Read the model definition and answer for the solid it produces. Units are mm, in the model's axes. A direction names the side the tool comes from. Round coordinates to 2 decimals unless told otherwise and drop trailing zeros. Order: outer loops, then holes, each group sorted by start corner. A loop starts at its lowest first (then second) coordinate and runs counter-clockwise, first axis right, second up. Notation, with made-up numbers: M 46,82.5 L 85,82.5 A32 ccw 85,116.5 Z; hole C 32.5,81.5 d2. An arc over 180 degrees is marked long. Use one line per item in the form item = value. Start each with the question number.
from build123d import *

# Parameters (mm, degrees)
SKETCH_3_W             = 8
SKETCH_3_H             = 16.823898374
CUT_EXTRUDE_1_DEPTH    = 10
HOLE_WIZARD_M4_1_D     = 3.3
HOLE_WIZARD_M4_1_DEPTH = 11.5
HOLE_WIZARD_M4_1_TIP   = 0.991420021
SKETCH_5_OUTSIDE_W     = 23.696
SKETCH_5_OUTSIDE_H     = 27.696
SKETCH_5_OUTSIDE_R     = 7.77784742
CUT_EXTRUDE_2_DEPTH    = 10


with BuildPart() as part:
    # 草图2 → 旋转1 (revolve)
    with BuildSketch(Plane(origin=(0, 0, 0), x_dir=(0, 0, -1), z_dir=(1, 0, 0))):
        Polygon((0, 0), (0, 4), (15, 4), (15, 9), (21, 9), (21, 4), (31, 4), (31, 0), align=None)
    revolve(axis=Axis((0, 0, 0), (0, 0, -1)))

    # 草图3 → 切除-拉伸1 (cut)
    with BuildSketch(Plane.XY.offset(-15)):
        with Locations((-11, -0.026043186)):
            Rectangle(SKETCH_3_W, SKETCH_3_H)
        with Locations((11, -0.026043186)):
            Rectangle(SKETCH_3_W, SKETCH_3_H)
    extrude(amount=-CUT_EXTRUDE_1_DEPTH, mode=Mode.SUBTRACT)

    # M4 螺纹孔1
    with Locations(Plane(origin=(0, 0, -31), x_dir=(-1, 0, 0), z_dir=(0, 0, -1))):
        with Locations((0, 0)):
            Hole(HOLE_WIZARD_M4_1_D / 2, depth=HOLE_WIZARD_M4_1_DEPTH)
            with Locations((0, 0, -(HOLE_WIZARD_M4_1_DEPTH + HOLE_WIZARD_M4_1_TIP / 2))):  # 118° drill point
                Cone(0, HOLE_WIZARD_M4_1_D / 2, HOLE_WIZARD_M4_1_TIP, mode=Mode.SUBTRACT)

    # 草图5 outside → 切除-拉伸2 (cut)
    with BuildSketch(Plane(origin=(0, 0, -21), x_dir=(-1, 0, 0), z_dir=(0, 0, -1))):
        Rectangle(SKETCH_5_OUTSIDE_W, SKETCH_5_OUTSIDE_H)
        Circle(SKETCH_5_OUTSIDE_R, mode=Mode.SUBTRACT)
    extrude(amount=-CUT_EXTRUDE_2_DEPTH, mode=Mode.SUBTRACT)


solid = part.part
Item 1: For a pull along Y with two mould halves and no side action, classify faces 1 (the conical face through (0.1, -0.3, -18.7)), 2 (the cylindrical face through (0.122, -7.777, -18.042)), 3 (the cylindrical face through (-3.905, -0.867, -7.605)) as pulls with the +Y half, pulls with the -Y half, needs draft (parallel to the pull), parting line crosses it, or undercut.
Item 2: Section B-B (x = 3.25) is taken. Write down the section's boundary in (y, z).
Item 3: Section A-A (z = -24) is taken. Write down the section's boundary in (x, y), and give its area (3 significant figures).
Item 4: Find the intervals of material crossed by L1, parallel to X at y = 0, z = -24.5; L2, parallel to Z at x = 4, y = -2.25; L3, parallel to Y at x = 0.5, z = -24, in increasing order. Write a range as [from, to].
Item 5: Section D-D (y = 6.75) is taken. Write down the section's boundary in (x, z).
Item 6: Given P1, Ø5, axis at x = -3, z = -27, coming from the -Y side; P2, Ø1, axis at x = 5, y = 1.5, coming from the -Z side; P3, Ø1.5, axis at y = 4, z = -26, coming from the +X side, each flat-ended and moving along its own axis, determine where each tip first touches the part or whether it passes through.
Item 7: Section C-C (z = -17) is taken. Write down the section's boundary in (x, y).
Item 8: A tool of negligible diameter and unlimited length cuts with its end or side. For faces 4 (the flat face through (0, 2, -31)), 5 (the flat face through (3, 4, -15)), 6 (the cylindrical face through (-3.905, -0.867, -26.07)), from which of +Z, -Z, +X, -X, +Y, -Y can it reach the whole face along a straight path? Write none if from no direction.
The answers:
q1.face_1 = undercut
q1.face_2 = pulls with the -Y half
q1.face_3 = parting line crosses it
q2.outline = M -7.07,-21 L -2.33,-21 L -2.33,-31 L 2.33,-31 L 2.33,-21 L 7.07,-21 L 7.07,-15 L 2.33,-15 L 2.33,0 L -2.33,0 L -2.33,-15 L -7.07,-15 Z
q3.outline = C 0,0 d8; hole C 0,0 d3.3
q3.area = 41.7 mm²
q4.L1 = [-4, -1.65], [1.65, 4]
q4.L2 = [-21, -15]
q4.L3 = [-3.97, -1.57], [1.57, 3.97]
q5.outline = M -3.86,-21 L 3.86,-21 L 3.86,-15 L -3.86,-15 Z
q6.P1 = -3.97
q6.P2 = -21
q6.P3 = 2.33
q7.outline = M -7,-3.39 A7.78 ccw 7,-3.39 L 7,3.39 A7.78 ccw -7,3.39 Z
q8.face_4 = -Z, +X, -X, +Y, -Y
q8.face_5 = +Z
q8.face_6 = -Z
